The model under review builds one solid part; all positions refer to its coordinate system, in mm. A direction names the side the tool comes from. Give positions to 0.01 mm unless a question says otherwise; leave off trailing zeros. Order: outer loops, then holes, each group sorted by start corner. A loop starts at its lowest first (then second) coordinate and runs counter-clockwise, first axis right, second up.
```python
from build123d import *

# Parameters (mm, degrees)
CROQUIS1_W              = 50.8
CROQUIS1_H              = 25.4
CROQUIS1_W_2            = 47.8
CROQUIS1_H_2            = 22.4
SALIENTE_EXTRUIR1_DEPTH = 400
CORTAR_EXTRUIR1_DEPTH   = 26


with BuildPart() as part:
    # Croquis1 → Saliente-Extruir1 (new body)
    with BuildSketch(Plane(origin=(0, 0, 0), x_dir=(1, 0, 0), z_dir=(0, 1, 0))):
        Rectangle(CROQUIS1_W, CROQUIS1_H)
        Rectangle(CROQUIS1_W_2, CROQUIS1_H_2, mode=Mode.SUBTRACT)
    extrude(amount=SALIENTE_EXTRUIR1_DEPTH)

    # Croquis2 → Cortar-Extruir1 (cut)
    with BuildSketch(Plane.XY.offset(12.7)):
        Polygon((-25.4, 0), (25.4, 50.8), (25.4, 0), align=None)
        Polygon((25.4, 400), (-25.4, 400), (25.4, 349.2), align=None)
    extrude(amount=-CORTAR_EXTRUIR1_DEPTH, mode=Mode.SUBTRACT)


solid = part.part
```
Item 1: Take a section at B-B (x = -2.5). Give the boundary of the cut face in (y, z), and give its area (3 significant figures).
Values found:
outline: (22.9, -12.7) - (377.1, -12.7) - (377.1, -11.2) - (22.9, -11.2) - close; (22.9, 11.2) - (377.1, 11.2) - (377.1, 12.7) - (22.9, 12.7) - close
area: 1,060 mm2
Item 2: For line 1 (X direction, y = 272, z = 8.75); line 2 (Z direction, x = -23, y = 356.5); line 3 (X direction, y = 356, z = -4), list the stretches that pass through material, from the lowest coordinate up.
Values found:
line 1: x = -25.4 to -23.9, 23.9 to 25.4
line 2: z = -12.7 to -11.2, 11.2 to 12.7
line 3: x = -25.4 to -23.9
Item 3: Draft analysis for pull direction Z (two halves, no side actions). For faces 3 (the flat face through (0, 197, -12.7)), 4 (the flat face through (-25.4, 197, 0)), 5 (the flat face through (0, 197, 11.2)), state which applies: released by +Z, released by -Z, zero draft, split by the parting line, or undercut.
Values found:
face 3: released by -Z
face 4: zero draft
face 5: undercut
Item 4: For faces 1 (the flat face through (23.9, 198, 0)), 2 (the flat face through (-0.1, 25.3, -12.2)), list the 3-axis set-ups (+Z, -Z, +X, -X, +Y, -Y) from which the entire face can be reached by the end or side of a thin tool; tool diameter is ignored.
Values found:
face 1: +Y, -Y
face 2: +Z, -Z, +X, -Y
Item 5: Take a section at D-D (y = 45.5). Give the boundary of the cut face in (x, z), and give its area (3 significant figures).
Values found:
outline: (-25.4, -12.7) - (20.1, -12.7) - (20.1, -11.2) - (-23.9, -11.2) - (-23.9, 11.2) - (20.1, 11.2) - (20.1, 12.7) - (-25.4, 12.7) - close
area: 170 mm2
Item 6: Take a section at C-C (y = 182). Give the boundary of the cut face in (x, z).
Values found:
outline: (-25.4, -12.7) - (25.4, -12.7) - (25.4, 12.7) - (-25.4, 12.7) - close; hole (-23.9, -11.2) - (23.9, -11.2) - (23.9, 11.2) - (-23.9, 11.2) - close
Item 7: Take a section at A-A (z = -4). Give the boundary of the cut face in (x, y), and give its area (3 significant figures).
Values found:
outline: (-25.4, 0) - (-23.9, 1.5) - (-23.9, 398.5) - (-25.4, 400) - close; (23.9, 49.3) - (25.4, 50.8) - (25.4, 349.2) - (23.9, 350.7) - close
area: 1,050 mm2
